Check sheet for the modelled part. Datum: model origin and axes. Units: mm. A direction names the side the tool comes from. Give positions to 0.01 mm unless a question says otherwise; leave off trailing zeros. Order: outer loops, then holes, each group sorted by start corner. A loop starts at its lowest first (then second) coordinate and runs counter-clockwise, first axis right, second up. Notation, with made-up numbers: (-2, 52.25) -> (24, 52.25) arc R25 ccw to (24, 73.25) -> close; hole circle Ø10 at (39.5, -11). An arc over 180 degrees is marked (long way). Write each question's results on one line, items separated by ' | '.
from build123d import *

# Parameters (mm, degrees)
F1_DEPTH      = 4
F1_DEPTH_BACK = 4
F0_W          = 16.4369798731
F0_H          = 6.529757753
F0_W_2        = 4.7284475295
F0_H_2        = 5.8542657644
F2_DEPTH      = 8.2
F2_DEPTH_BACK = 11.1
F3_DEPTH      = 4.1
F3_DEPTH_BACK = 8.9
F0_W_3        = 13.7350079603
F0_H_3        = 3.3774608746
F4_DEPTH      = 4.9
F4_DEPTH_BACK = 6.6
F5_R          = 5


with BuildPart() as f1:
    # F0 (on Front) → F1 (new body, two sides)
    with BuildSketch(Plane.XZ) as f1_sk:
        Polygon((10.553249158, 21.6060578823), (2.897671191, 21.6060578823), (2.897671191, 15.0763001293), (-13.5393086821, 15.0763001293), (-13.5393086821, -12.6188807189), (-9.2611899599, -12.6188807189), (-9.2611899599, -9.2414198443), (4.4738180004, -9.2414198443), (4.4738180004, -12.6188807189), (10.553249158, -12.6188807189), align=None)
    extrude(amount=F1_DEPTH)
    extrude(f1_sk.sketch, amount=-F1_DEPTH_BACK)

    # F0 (on Front) → F2 (join, two sides)
    with BuildSketch(Plane.XZ) as f2_sk:
        with Locations((-5.3208187455, 18.3411790058)):
            Rectangle(F0_W, F0_H)
        Polygon((-13.5393086821, 15.0763001293), (-13.5393086821, 21.6060578823), (2.897671191, 21.6060578823), (2.897671191, 26.784831658), (-1.8307763385, 26.784831658), (-1.8307763385, 32.6390974224), (-23.6716903746, 32.6390974224), (-23.6716903746, 15.0763001293), align=None)
        with Locations((0.5334474263, 29.7119645402)):
            Rectangle(F0_W_2, F0_H_2)
    extrude(amount=F2_DEPTH)
    extrude(f2_sk.sketch, amount=-F2_DEPTH_BACK)

    # F0 (on Front) → F3 (join, two sides)
    with BuildSketch(Plane.XZ) as f3_sk:
        Polygon((2.897671191, 32.6390974224), (2.897671191, 26.784831658), (13.9307100326, 26.784831658), (13.9307100326, 40.7450050116), (-1.8307763385, 40.7450050116), (-1.8307763385, 32.6390974224), align=None)
        with Locations((0.5334474263, 29.7119645402)):
            Rectangle(F0_W_2, F0_H_2)
    extrude(amount=F3_DEPTH)
    extrude(f3_sk.sketch, amount=-F3_DEPTH_BACK)

    # F0 (on Front) → F4 (join, two sides)
    with BuildSketch(Plane.XZ) as f4_sk:
        with Locations((-2.3936859798, -10.9301502816)):
            Rectangle(F0_W_3, F0_H_3)
        with Locations((-2.3936859798, -15.8837595955)):
            Rectangle(F0_W_3, F0_H)
    extrude(amount=F4_DEPTH)
    extrude(f4_sk.sketch, amount=-F4_DEPTH_BACK)

    # F5
    f5_edges = [f1.edges().sort_by_distance(p)[0] for p in [
        (10.553249, 4, 4.493589),
        (-9.26119, -4.9, -14.195029),
    ]]
    fillet(f5_edges, radius=F5_R)


solid = f1.part
1. Gauge pin test, flat ends, axial feed: pin 1 Ø9.5 at (x, z) = (-0.5, -15) entering from -Y; pin 2 Ø5 at (x, z) = (3, -2.5) entering from -Y; pin 3 Ø11 at (y, z) = (3, -15.5) entering from +X. Record the tip position at first contact, or that the pin passes through.
Verdict:
pin 1: stops at y = -4.9 | pin 2: stops at y = -4 | pin 3: stops at x = 10.55
2. Section check A-A on x = 0.5. Record the cut outline in (y, z) (3 decimals), then the cut area to 3 significant figures.
Verdict:
outline: (-8.2, 15.076) -> (-4, 15.076) -> (-4, -9.241) -> (-4.9, -9.241) -> (-4.9, -19.149) -> (6.6, -19.149) -> (6.6, -9.241) -> (4, -9.241) -> (4, 15.076) -> (11.1, 15.076) -> (11.1, 32.639) -> (8.9, 32.639) -> (8.9, 40.745) -> (-4.1, 40.745) -> (-4.1, 32.639) -> (-8.2, 32.639) -> close | area: 753 mm^2
3. Section check D-D on x = 7.5. Record the cut outline in (y, z) (3 decimals), then the cut area to 3 significant figures.
Verdict:
outline: (-4.1, 26.785) -> (8.9, 26.785) -> (8.9, 40.745) -> (-4.1, 40.745) -> close; (-4, -12.619) -> (3.605, -12.619) -> (3.605, 21.606) -> (-4, 21.606) -> close | area: 442 mm^2
4. Material ranges on probe 1 along X at (y, z) = (8, 18); probe 2 along Z at (x, y) = (-21.5, -6.25); probe 3 along Z at (x, y) = (-5, 2.75), recorded low to high. Write a range as from..to.
Verdict:
probe 1: x = -23.67..2.9 | probe 2: z = 15.08..32.64 | probe 3: z = -19.15..32.64
5. Section check C-C on y = -7. Record the cut outline in (x, z), then the cut area to 3 significant figures.
Verdict:
outline: (-23.67, 15.08) -> (2.9, 15.08) -> (2.9, 32.64) -> (-23.67, 32.64) -> close | area: 467 mm^2
6. Access from +Z, -Z, +X, -X, +Y, -Y to the whole of each face (thin tool, end or side, straight path). Record for faces 1 (the flat face through (7, 0, 21.606)), 2 (the flat face through (-13.539, 0, 1)), 3 (the cylindrical face through (9.127, 2.496, 4.733)), 4 (the flat face through (-1.831, 2, 37)).
Verdict:
face 1: +X, +Y, -Y | face 2: -Z, -X, +Y, -Y | face 3: -Z, +X, +Y | face 4: +Z, -X, +Y, -Y
7. Section check B-B on z = 29. Record the cut outline in (x, y).
Verdict:
outline: (-23.67, -8.2) -> (2.9, -8.2) -> (2.9, -4.1) -> (13.93, -4.1) -> (13.93, 8.9) -> (2.9, 8.9) -> (2.9, 11.1) -> (-23.67, 11.1) -> close
8. Mould release check, pull along Z, two halves, no side actions. Record for faces 5 (the flat face through (7, 0, -12.619)), 6 (the flat face through (-4, 4, 5)), 7 (the flat face through (8, -4.1, 34)): +Z half, -Z half, draft (parallel to the pull), parting line (faces both ways), or undercut.
Verdict:
face 5: -Z half | face 6: undercut | face 7: draft
